```python
from build123d import *

# Parameters (mm, degrees)
EXTRUDE_DEPTH  = 5
BOX019_W       = 530
BOX019_H       = 5
BOX019_DEPTH   = 200
BOX020_W       = 530
BOX020_H       = 5
BOX020_DEPTH   = 200
BOX021_W       = 520
BOX021_H       = 500
BOX021_DEPTH   = 250
THICKNESS001_T = 10


with BuildPart() as extrude_body:
    # Sketch (on Face43 of Cut004) → Extrude (new body)
    with BuildSketch(Plane(origin=(0, 0, -63.6), x_dir=(1, 0, 0), z_dir=(0, 0, -1))):
        with BuildLine():
            Line((20, -235), (500, -235))
            ThreePointArc((500, -265), (515, -250), (500, -235))
            Line((20, -265), (500, -265))
            ThreePointArc((20, -235), (5, -250), (20, -265))
        make_face()
    extrude(amount=-EXTRUDE_DEPTH)


with BuildPart() as supportrail003:
    # Box019 → Box019 (new body)
    with BuildSketch(Plane(origin=(-5.7935, 85.5, 13.6), x_dir=(1, 0, 0), z_dir=(0, 0, 1))):
        with Locations((265, 2.5)):
            Rectangle(BOX019_W, BOX019_H)
    extrude(amount=BOX019_DEPTH)


with BuildPart() as supportrail004:
    # Box020 → Box020 (new body)
    with BuildSketch(Plane(origin=(-5.7935, 454, 17.5), x_dir=(1, 0, 0), z_dir=(0, 0, 1))):
        with Locations((265, 2.5)):
            Rectangle(BOX020_W, BOX020_H)
    extrude(amount=BOX020_DEPTH)


with BuildPart() as box:
    # Box021 → Box021 (new body)
    with BuildSketch(Plane.XY):
        with Locations((260, 250)):
            Rectangle(BOX021_W, BOX021_H)
    extrude(amount=BOX021_DEPTH)

    # Thickness001
    thickness001_openings = [box.faces().sort_by_distance(p)[0] for p in [
        (260, 250, 250),
    ]]
    offset(amount=THICKNESS001_T, openings=thickness001_openings)

    # Cut003: cut SupportRail004
    add(supportrail004.part, mode=Mode.SUBTRACT)

    # Cut004: cut SupportRail003
    add(supportrail003.part, mode=Mode.SUBTRACT)


with BuildPart() as box_1:
    # Cut004 placement: moved
    add(box.part.moved(Location((0, 0, -53.6))))

    # Cut005: cut Extrude body
    add(extrude_body.part, mode=Mode.SUBTRACT)


solid = box_1.part
```
Build history of the part. All positions in model axes, mm. A direction names the side the tool comes from. Give positions to 0.01 mm unless a question says otherwise; leave off trailing zeros. Order: outer loops, then holes, each group sorted by start corner. A loop starts at its lowest first (then second) coordinate and runs counter-clockwise, first axis right, second up. Notation, with made-up numbers: M 82.25,11 L 119.25,11 A23 ccw 119.25,44 Z; hole C -35.5,22.25 d8. An arc over 180 degrees is marked long. Return JSON: item names as keys, results as strings.
Q1. Band-saw the part on B-B (x = 172). Give the cut face in (y, z), then the cut area to 3 significant figures.
Answer list:
{"outline": "M -10,-53.6 A10 ccw 0,-63.6 L 235,-63.6 L 235,-58.6 L 265,-58.6 L 265,-63.6 L 500,-63.6 A10 ccw 510,-53.6 L 510,196.4 L 500,196.4 L 500,-53.6 L 0,-53.6 L 0,196.4 L -10,196.4 Z", "area": "10,000 mm^2"}
Q2. Band-saw the part on C-C (y = 250). Give the cut face in (x, z).
Answer list:
{"outline": "M -10,-53.6 A10 ccw 0,-63.6 L 5,-63.6 L 5,-58.6 L 515,-58.6 L 515,-63.6 L 520,-63.6 A10 ccw 530,-53.6 L 530,196.4 L 520,196.4 L 520,-53.6 L 0,-53.6 L 0,196.4 L -10,196.4 Z"}
Q3. Two-plate mould, pull along X, no slides. Class faces 1 (the face through (5, 250, -61)), 2 (the face through (-10, 247, 70)), 3 (the face through (256, 510, 70)): pulls with the +X half, pulls with the -X half, needs draft (parallel to the pull), parting line crosses it, or undercut.
Answer list:
{"face 1": "undercut", "face 2": "pulls with the -X half", "face 3": "needs draft"}
Q4. Wall check: probe 1 along X at (y, z) = (177, 87); probe 2 along Y at (x, z) = (358, 26.5); probe 3 along Z at (x, y) = (102, 115.5). Give the ranges that are in metal, low to high. Write a range as from..to.
Answer list:
{"probe 1": "x = -10..0, 520..530", "probe 2": "y = -10..0, 500..510", "probe 3": "z = -63.6..-53.6"}
Q5. Flat gauge pins, fed straight in: pin 1 (5.5 mm diameter, centred on x = 219.5, z = -61.5, fed in from +Y); pin 2 (1.7 mm diameter, centred on x = -3.5, z = 66.5, fed in from +Y); pin 3 (4 mm diameter, centred on x = -3.5, y = 456, fed in from -Z); pin 4 (4.5 mm diameter, centred on x = -2, z = 113.5, fed in from -Y). Where does each tip first touch, or does it go through?
Answer list:
{"pin 1": "stops at y = 508.57", "pin 2": "stops at y = 509.64", "pin 3": "stops at z = -63.49", "pin 4": "stops at y = -10"}
Q6. Band-saw the part on A-A (z = -21). Give the cut face in (x, y), then the cut area to 3 significant figures.
Answer list:
{"outline": "M -10,0 A10 ccw 0,-10 L 520,-10 A10 ccw 530,0 L 530,500 A10 ccw 520,510 L 0,510 A10 ccw -10,500 Z; hole M -5.79,85.5 L 0,85.5 L 0,0 L 520,0 L 520,85.5 L 524.21,85.5 L 524.21,90.5 L 520,90.5 L 520,454 L 524.21,454 L 524.21,459 L 520,459 L 520,500 L 0,500 L 0,459 L -5.79,459 L -5.79,454 L 0,454 L 0,90.5 L -5.79,90.5 Z", "area": "20,600 mm^2"}
Q7. 3-axis set-ups, long thin cutter, end or side, ignore diameter. For faces 4 (the face through (256, 500, 70)), 5 (the face through (264, 250, -58.6)), 6 (the face through (139, 502, 196.4)): which of +Z, -Z, +X, -X, +Y, -Y reach the whole face in a straight line?
Answer list:
{"face 4": "+Z", "face 5": "-Z", "face 6": "+Z, +X, -X, +Y, -Y"}
Q8. Band-saw the part on D-D (y = 38). Give the cut face in (x, z).
Answer list:
{"outline": "M -10,-53.6 A10 ccw 0,-63.6 L 520,-63.6 A10 ccw 530,-53.6 L 530,196.4 L 520,196.4 L 520,-53.6 L 0,-53.6 L 0,196.4 L -10,196.4 Z"}
